Can you work these out from the model? Positions are in its coordinate system, mm. Coordinates: 2 decimals unless noted, no trailing zeros. Write each loop counter-clockwise with the first axis right and the second up, starting at its lowest first coordinate (ties: lowest second). Pieces come first, ordered by that corner, then holes.
```python
from build123d import *

# Parameters (mm, degrees)
F1_DEPTH = 203.2
F1_TAPER = 1
F2_DEPTH = 25.4
F2_TAPER = 25
F3_SIZE  = 11.43


with BuildPart() as f1:
    # F0 (on Top) → F1 (new body)
    with BuildSketch(Plane.XY):
        Polygon((0, 12.7), (-38.1, 0), (0, -12.7), (38.1, 0), align=None)
    extrude(amount=F1_DEPTH, taper=F1_TAPER)

    # F1_face (on face) → F2 (join)
    with BuildSketch(Plane.XY.offset(203.2)):
        Polygon((0, 8.9612715954), (-26.8838147861, 0), (0, -8.9612715954), (26.8838147861, 0), align=None)
    extrude(amount=F2_DEPTH, taper=F2_TAPER)

    # F3
    f3_edges = [f1.edges().sort_by_distance(p)[0] for p in [
        (-19.05, 6.35, 0),
        (19.05, 6.35, 0),
        (19.05, -6.35, 0),
        (-19.05, -6.35, 0),
    ]]
    chamfer(f3_edges, length=F3_SIZE)


solid = f1.part
```
1. If we section it at A-A, the plane y = 3.25: List the corners of the cut face in (x, z) for me.
2. If we section it at B-B, the plane x = 9.5: List the corners of the cut face in (y, z) for me, plus the area to 3 significant figures.
3. If we section it at C-C, the plane z = 51: List the corners of the cut face in (x, y) for me.
4. If I drill on L1, parallel to Y at x = 15.5, z = 18; L2, parallel to Y at x = -26.5, z = 34; L3, parallel to Z at x = -16, y = -3.5, over which ranges is the centre line in solid material (lowest first)?
5. If we section it at D-D, the plane z = 94: List the corners of the cut face in (x, y) for me, plus the area to 3 significant figures.
6. I'm going to push flat-ended pins straight in: P1, Ø1, axis at y = -10, z = 194, coming from the -X side; P2, Ø2, axis at x = 23.5, y = -2, coming from the +Z side; P3, Ø6, axis at x = 10, z = 119, coming from the -Y side; P4, Ø3, axis at x = -14, z = 101.5, coming from the -Y side. Where does each tip first touch, or does it pass through?
Answers:
1. outline: (-27.72, 11.43) - (0, 2.51) - (27.72, 11.43) - (17.13, 203.2) - (0, 214.82) - (-17.13, 203.2) - close
2. outline: (-9.32, 11.43) - (0, 2.43) - (9.32, 11.43) - (5.79, 203.2) - (0, 214.99) - (-5.79, 203.2) - close
2. area: 3,050 mm2
3. outline: (-35.28, 0) - (0, -11.76) - (35.28, 0) - (0, 11.76) - close
4. L1: y = -7.2 to 7.2
4. L2: y = -3.24 to 3.24
4. L3: z = 7.9 to 203.46
5. outline: (-32.91, 0) - (0, -10.97) - (32.91, 0) - (0, 10.97) - close
5. area: 722 mm2
6. P1: passes through
6. P2: stops at z = 203.57
6. P3: stops at y = -8.18
6. P4: stops at y = -6.67
